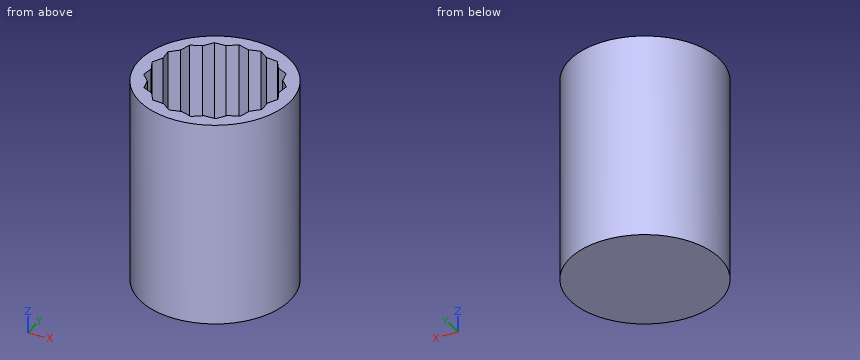
from build123d import *

# Parameters (mm, degrees)
SKETCH_R           = 3.65
PAD_DEPTH          = 10
POCKET_DEPTH       = 8
POLARPATTERN_COUNT = 18


with BuildPart() as part:
    # Sketch → Pad (new body)
    with BuildSketch(Plane.XY):
        Circle(SKETCH_R)
    extrude(amount=PAD_DEPTH)

    # Sketch001 (on Face3 of Pad) → Pocket (cut)
    with BuildSketch(Plane.XY.offset(10)):
        Polygon((-2.9130471244, 1.0602624443), (0, 0), (-3.1, 0), (-2.8559424837, 0.5035797152), align=None)
    pocket = extrude(amount=-POCKET_DEPTH, mode=Mode.SUBTRACT)

    # PolarPattern: Pocket ×18 about axis
    polarpattern_axis = Axis((0, 0, 10), (0, 0, 1))
    for i in range(1, POLARPATTERN_COUNT):
        add(pocket.rotate(polarpattern_axis, i * 360 / POLARPATTERN_COUNT), mode=Mode.SUBTRACT)


solid = part.part
Verification items for the finished model (mm, model axes). Coordinates: 2 decimals unless noted, no trailing zeros. Write each loop counter-clockwise with the first axis right and the second up, starting at its lowest first coordinate (ties: lowest second). Pieces come first, ordered by that corner, then holes. Notation, with made-up numbers: M 35,25.5 L 59,25.5 A22 ccw 59,41.5 Z; hole C 46.5,16.25 d6. An arc over 180 degrees is marked long. One line per question, with ' | ' between items.
1) Depth check by flat-ended pin: pin 1 Ø2 at (x, y) = (1, -0.5) entering from +Z; pin 2 Ø2 at (x, y) = (-2, 1) entering from +Z; pin 3 Ø1 at (y, z) = (-2.5, 9) entering from +X; pin 4 Ø2 at (y, z) = (-1.5, 1.5) entering from -X. Enter the tip coordinate at first touch or a pass-through.
Solutions:
pin 1: z = 2 | pin 2: z = 10 | pin 3: x = 3.05 | pin 4: x = -3.62
2) Material ranges on L1, parallel to Z at x = 0.25, y = 2.25; L2, parallel to Y at x = -1.5, z = 3.75; L3, parallel to X at y = 2.5, z = 5.5, recorded low to high.
Solutions:
L1: 0 to 2 | L2: -3.33 to -2.69, 2.69 to 3.33 | L3: -2.66 to -1.68, 1.68 to 2.66
3) Sectioned sample at A-A on x = -2.25. Record the cut outline in (y, z), then the cut area to 3 significant figures.
Solutions:
outline: M -2.87,0 L 2.87,0 L 2.87,10 L 2.05,10 L 2.05,2 L -2.05,2 L -2.05,10 L -2.87,10 Z | area: 24.7 mm^2
4) Sectioned sample at B-B on y = -2.5. Record the cut outline in (x, z), then the cut area to 3 significant figures.
Solutions:
outline: M -2.66,0 L 2.66,0 L 2.66,10 L 1.68,10 L 1.68,2 L -1.68,2 L -1.68,10 L -2.66,10 Z | area: 26.4 mm^2
5) Sectioned sample at C-C on z = 1.75. Record the cut outline in (x, y), then the cut area to 3 significant figures.
Solutions:
outline: C 0,0 d7.3 | area: 41.9 mm^2
